Design review of the part built by this model. Coordinates are the model's own, in mm. A direction names the side the tool comes from. Coordinates: 2 decimals unless noted, no trailing zeros. Write each loop counter-clockwise with the first axis right and the second up, starting at its lowest first coordinate (ties: lowest second). Pieces come first, ordered by that corner, then holes. Notation, with made-up numbers: M 55.5,54.25 L 60.5,54.25 A19 ccw 60.5,91.25 Z; hole C -28.5,-25.5 d10. An arc over 180 degrees is marked long. One line per question, with ' | ' between items.
from build123d import *

# Parameters (mm, degrees)
BOSS_EXTRUDE4_DEPTH = 200
SKETCH5_W           = 300
SKETCH5_H           = 140
CUT_EXTRUDE3_DEPTH  = 270
SKETCH6_W           = 2.411871081
SKETCH6_H           = 3
SKETCH6_W_2         = 30
SKETCH6_W_3         = 2.243969638
SKETCH6_W_4         = 1.678083374
SKETCH6_W_5         = 1.954362123
BOSS_EXTRUDE6_DEPTH = 200
SKETCH7_W           = 100
SKETCH7_H           = 140
CUT_EXTRUDE4_DEPTH  = 174
SKETCH9_W           = 50
SKETCH9_H           = 30
BOSS_EXTRUDE7_DEPTH = 193
SKETCH10_R          = 12.5
CUT_EXTRUDE5_DEPTH  = 193
CUT_EXTRUDE23_DEPTH = 10


with BuildPart() as part:
    # Sketch1 → Boss-Extrude4 (new body)
    with BuildSketch(Plane.XY):
        Polygon((1.862238879, 123.981049527), (1.862238879, 153.981049527), (-33.137761121, 153.981049527), (-133.137761121, 3.981049527), (-133.137761121, -146.018950473), (-53.137761121, -146.018950473), (86.862238879, -146.018950473), (166.862238879, -146.018950473), (166.862238879, 3.981049527), (66.862238879, 153.981049527), (31.862238879, 153.981049527), (31.862238879, 123.981049527), (50.806726124, 123.981049527), (136.862238879, -5.102219605), (136.862238879, -116.018950473), (31.862238879, -116.018950473), (31.862238879, -46.018950473), (1.862238879, -46.018950473), (1.862238879, -116.018950473), (-103.137761121, -116.018950473), (-103.137761121, -5.102219605), (-17.082248367, 123.981049527), align=None)
        Polygon((31.862238879, 153.981049527), (1.862238879, 153.981049527), (1.862238879, 123.981049527), (1.862238879, -46.018950473), (31.862238879, -46.018950473), (31.862238879, 123.981049527), align=None)
    extrude(amount=BOSS_EXTRUDE4_DEPTH)

    # Sketch5 → Cut-Extrude3 (cut)
    with BuildSketch(Plane.XZ.offset(146.018950473)):
        with Locations((16.862238879, 100)):
            Rectangle(SKETCH5_W, SKETCH5_H)
    extrude(amount=-CUT_EXTRUDE3_DEPTH, mode=Mode.SUBTRACT)

    # Sketch6 → Boss-Extrude6 (add)
    with BuildSketch(Plane.XY.offset(200)):
        with Locations((-134.343696662, -79.518950473)):
            Rectangle(SKETCH6_W, SKETCH6_H)
        with Locations((-118.137761121, -79.518950473)):
            Rectangle(SKETCH6_W_2, SKETCH6_H)
        with Locations((-102.015776302, -79.518950473)):
            Rectangle(SKETCH6_W_3, SKETCH6_H)
        with Locations((151.862238879, -79.518950473)):
            Rectangle(SKETCH6_W_2, SKETCH6_H)
        with Locations((167.701280566, -79.518950473)):
            Rectangle(SKETCH6_W_4, SKETCH6_H)
        with Locations((135.885057818, -79.518950473)):
            Rectangle(SKETCH6_W_5, SKETCH6_H)
    extrude(amount=-BOSS_EXTRUDE6_DEPTH)

    # Sketch7 → Cut-Extrude4 (cut)
    with BuildSketch(Plane(origin=(0, 153.981049527, 0), x_dir=(1, 0, 0), z_dir=(0, 1, 0))):
        with Locations((16.862238879, -100)):
            Rectangle(SKETCH7_W, SKETCH7_H)
    extrude(amount=-CUT_EXTRUDE4_DEPTH, mode=Mode.SUBTRACT)

    # Sketch9 → Boss-Extrude7 (add)
    with BuildSketch(Plane(origin=(0, 0, 0), x_dir=(-1, 0, 0), z_dir=(0, 0, -1))):
        with Locations((-16.862238879, -131.018950473)):
            Rectangle(SKETCH9_W, SKETCH9_H)
    extrude(amount=-BOSS_EXTRUDE7_DEPTH)

    # Sketch10 → Cut-Extrude5 (cut)
    with BuildSketch(Plane.XZ.offset(146.018950473)):
        with Locations((16.862238879, 100)):
            Circle(SKETCH10_R)
    extrude(amount=-CUT_EXTRUDE5_DEPTH, mode=Mode.SUBTRACT)

    # Sketch11 → Cut-Extrude23 (cut)
    with BuildSketch(Plane(origin=(0, -78.018950473, 0), x_dir=(1, 0, 0), z_dir=(0, 1, 0))):
        with BuildLine():
            Line((139.362238879, -125.5), (143.362238879, -125.5))
            ThreePointArc((143.362238879, -125.5), (145.362238879, -127.5), (143.362238879, -129.5))
            Line((143.362238879, -129.5), (139.362238879, -129.5))
            ThreePointArc((139.362238879, -129.5), (137.362238879, -127.5), (139.362238879, -125.5))
        make_face()
        with BuildLine():
            Line((164.362238879, -125.5), (160.362238879, -125.5))
            ThreePointArc((160.362238879, -125.5), (158.362238879, -127.5), (160.362238879, -129.5))
            Line((160.362238879, -129.5), (164.362238879, -129.5))
            ThreePointArc((164.362238879, -129.5), (166.362238879, -127.5), (164.362238879, -125.5))
        make_face()
        with BuildLine():
            Line((164.362238879, -74.5), (160.362238879, -74.5))
            ThreePointArc((160.362238879, -74.5), (158.362238879, -72.5), (160.362238879, -70.5))
            Line((160.362238879, -70.5), (164.362238879, -70.5))
            ThreePointArc((164.362238879, -70.5), (166.362238879, -72.5), (164.362238879, -74.5))
        make_face()
        with BuildLine():
            Line((139.362238879, -74.5), (143.362238879, -74.5))
            ThreePointArc((143.362238879, -74.5), (145.362238879, -72.5), (143.362238879, -70.5))
            Line((143.362238879, -70.5), (139.362238879, -70.5))
            ThreePointArc((139.362238879, -70.5), (137.362238879, -72.5), (139.362238879, -74.5))
        make_face()
        with BuildLine():
            Line((-130.637761121, -125.5), (-126.637761121, -125.5))
            ThreePointArc((-126.637761121, -125.5), (-124.637761121, -127.5), (-126.637761121, -129.5))
            Line((-126.637761121, -129.5), (-130.637761121, -129.5))
            ThreePointArc((-130.637761121, -129.5), (-132.637761121, -127.5), (-130.637761121, -125.5))
        make_face()
        with BuildLine():
            Line((-105.637761121, -125.5), (-109.637761121, -125.5))
            ThreePointArc((-109.637761121, -125.5), (-111.637761121, -127.5), (-109.637761121, -129.5))
            Line((-109.637761121, -129.5), (-105.637761121, -129.5))
            ThreePointArc((-105.637761121, -129.5), (-103.637761121, -127.5), (-105.637761121, -125.5))
        make_face()
        with BuildLine():
            Line((-130.637761121, -74.5), (-126.637761121, -74.5))
            ThreePointArc((-126.637761121, -74.5), (-124.637761121, -72.5), (-126.637761121, -70.5))
            Line((-126.637761121, -70.5), (-130.637761121, -70.5))
            ThreePointArc((-130.637761121, -70.5), (-132.637761121, -72.5), (-130.637761121, -74.5))
        make_face()
        with BuildLine():
            Line((-105.637761121, -74.5), (-109.637761121, -74.5))
            ThreePointArc((-109.637761121, -74.5), (-111.637761121, -72.5), (-109.637761121, -70.5))
            Line((-109.637761121, -70.5), (-105.637761121, -70.5))
            ThreePointArc((-105.637761121, -70.5), (-103.637761121, -72.5), (-105.637761121, -74.5))
        make_face()
    extrude(amount=-CUT_EXTRUDE23_DEPTH, mode=Mode.SUBTRACT)


solid = part.part
1. Insertion check: pin 1 Ø10 at (x, z) = (-97.5, 144.5) entering from -Y; pin 2 Ø15 at (y, z) = (-102.5, 184.5) entering from +X; pin 3 Ø9 at (y, z) = (137, 106.5) entering from +X; pin 4 Ø6 at (x, y) = (122.5, 7) entering from -Z. Each pin has a flat end and moves straight along its axis. Give the tip position at first contact, or say it passes through.
Answer sheet:
pin 1: y = -81.02 | pin 2: x = 166.86 | pin 3: x = 81.18 | pin 4: through
2. Take a section at C-C (x = -12.5). Write out the cut boundary in (y, z).
Answer sheet:
outline: M -146.02,0 L -116.02,0 L -116.02,30 L -146.02,30 Z; M -146.02,170 L -116.02,170 L -116.02,200 L -146.02,200 Z; M 123.98,0 L 153.98,0 L 153.98,30 L 123.98,30 Z; M 123.98,170 L 153.98,170 L 153.98,200 L 123.98,200 Z
3. Take a section at B-B (z = 49.5). Write out the cut boundary in (x, y).
Answer sheet:
outline: M -135.55,-81.02 L -100.89,-81.02 L -100.89,-78.02 L -135.55,-78.02 Z; M -53.14,123.98 L -33.14,123.98 L -33.14,153.98 Z; M -8.14,-146.02 L 41.86,-146.02 L 41.86,-116.02 L -8.14,-116.02 Z; M 66.86,123.98 L 86.86,123.98 L 66.86,153.98 Z; M 134.91,-81.02 L 168.54,-81.02 L 168.54,-78.02 L 134.91,-78.02 Z
4. Tool access review of faces 1 (the face through (117, -128, 30)), 2 (the face through (-85, -128, 30)), 3 (the face through (9, -116.019, 85)), 4 (the face through (41.862, -131, 99)), 5 (the face through (-103.138, -42, 15)): name each direction out of +Z, -Z, +X, -X, +Y, -Y from which nothing blocks a thin tool from reaching the whole face with its end or side.
Answer sheet:
face 1: +X, -Y | face 2: -X, -Y | face 3: none | face 4: +X, +Y, -Y | face 5: +Z, -Z
5. Draft analysis for pull direction Z (two halves, no side actions). For faces 6 (the face through (166.862, -38, 15)), 7 (the face through (77, 123.981, 101)), 8 (the face through (14, -27, 200)), state which applies: pulls with the +Z half, pulls with the -Z half, needs draft (parallel to the pull), parting line crosses it, or undercut.
Answer sheet:
face 6: needs draft | face 7: undercut | face 8: pulls with the +Z half
6. To check wall thickness, follow line 1 along Z through (x, y) = (-75.5, 77.5); line 2 along Y through (x, z) = (-6.5, 27); line 3 along X through (y, z) = (1, 183). State the ranges of each line that lie inside material, in increasing order. Write a range as [from, to].
Answer sheet:
line 1: [0, 30], [170, 200] | line 2: [-146.02, -116.02], [123.98, 153.98] | line 3: [-133.14, -99.07], [1.86, 31.86], [132.79, 166.86]
7. Take a section at D-D (z = 100). Write out the cut boundary in (x, y).
Answer sheet:
outline: M -135.55,-81.02 L -100.89,-81.02 L -100.89,-78.02 L -135.55,-78.02 Z; M -53.14,123.98 L -33.14,123.98 L -33.14,153.98 Z; M -8.14,-146.02 L 4.36,-146.02 L 4.36,-116.02 L -8.14,-116.02 Z; M 29.36,-146.02 L 41.86,-146.02 L 41.86,-116.02 L 29.36,-116.02 Z; M 66.86,123.98 L 86.86,123.98 L 66.86,153.98 Z; M 134.91,-81.02 L 168.54,-81.02 L 168.54,-78.02 L 134.91,-78.02 Z
8. Take a section at A-A (y = -101). Write out the cut boundary in (x, z), then the cut area to 3 significant figures.
Answer sheet:
outline: M -133.14,0 L -103.14,0 L -103.14,30 L -133.14,30 Z; M -133.14,170 L -103.14,170 L -103.14,200 L -133.14,200 Z; M 1.86,0 L 31.86,0 L 31.86,30 L 1.86,30 Z; M 1.86,170 L 31.86,170 L 31.86,200 L 1.86,200 Z; M 136.86,0 L 166.86,0 L 166.86,30 L 136.86,30 Z; M 136.86,170 L 166.86,170 L 166.86,200 L 136.86,200 Z | area: 5,400 mm^2
